Work out the finished part from the listing and answer in its coordinate system (mm). Round coordinates to 2 decimals unless told otherwise and drop trailing zeros. Write each loop counter-clockwise with the first axis right and the second up, starting at its lowest first coordinate (ties: lowest second). Pieces come first, ordered by that corner, then holes.
1. Find section B-B (y = 8.89). Write down the section's boundary in (x, z), and give its area (3 significant figures).
2. Find section A-A (y = -8.89). Write down the section's boundary in (x, z), and give its area (3 significant figures).
3. Determine the mould class of faces 1 (the face through (39.2, -15.4, 0.8)), 2 (the face through (-20.56, -7.94, 4.37)), 3 (the face through (-22, -10, 4.5)) for opening direction X: pulls with the +X half, pulls with the -X half, needs draft (parallel to the pull), parting line crosses it, or undercut.
4. Find section D-D (x = -16). Write down the section's boundary in (y, z), and give its area (3 significant figures).
5. Find section C-C (z = 3.6). Write down the section's boundary in (x, y), and give its area (3 significant figures).
6. A flat-ended cylindrical pin translates along its axis: pin 1 Ø4 at (x, y) = (36.51, -12.7) entering from +Z. Find the tip coordinate at first contact, or state that the pin passes through.
7. Straight lines are drawn through the part: probe 1 along X at (y, z) = (-8.5, 0.4); probe 2 along X at (y, z) = (-9.5, 4.2); probe 3 along Z at (x, y) = (30, -11). For each, find the intervals that lie inside material, in ascending order.
Autodesk Fusion 360 part; units mm, degrees
sketch "Sketch1" plane through (0, 0, 0) normal (0, 0, 1) x (1, 0, 0)
  line L0 (36.5125, -12.7) -> (-36.5125, -12.7) construction
  line L1 (-36.5125, -12.7) -> (-36.5125, 12.7) construction
  line L2 (-36.5125, 12.7) -> (36.5125, 12.7) construction
  line L3 (36.5125, 12.7) -> (36.5125, -12.7) construction
  line L4 (36.5125, -12.7) -> (-36.5125, 12.7) construction
  line L5 (-36.5125, -12.7) -> (36.5125, 12.7) construction
  line L6 (40.3225, -16.51) -> (-40.3225, -16.51)
  line L7 (-40.3225, -16.51) -> (-40.3225, 16.51)
  line L8 (-40.3225, 16.51) -> (40.3225, 16.51)
  line L9 (40.3225, 16.51) -> (40.3225, -16.51)
  circle A0 centre (-36.5125, 12.7) radius 1.524
  circle A1 centre (36.5125, 12.7) radius 1.524
  circle A2 centre (-36.5125, -12.7) radius 1.524
  circle A3 centre (36.5125, -12.7) radius 1.524
  line L10 (22.86, -8.89) -> (-22.86, -8.89) construction
  line L11 (-22.86, -8.89) -> (-22.86, 8.89) construction
  line L12 (-22.86, 8.89) -> (22.86, 8.89) construction
  line L13 (22.86, 8.89) -> (22.86, -8.89) construction
  line L14 (22.86, -8.89) -> (-22.86, 8.89) construction
  line L15 (-22.86, -8.89) -> (22.86, 8.89) construction
  circle A4 centre (-22.86, 8.89) radius 1.143
  circle A5 centre (22.86, 8.89) radius 1.143
  circle A6 centre (-22.86, -8.89) radius 1.143
  circle A7 centre (22.86, -8.89) radius 1.143
  circle A8 centre (-22.86, 8.89) radius 2.413
  circle A9 centre (22.86, 8.89) radius 2.413
  circle A10 centre (-22.86, -8.89) radius 2.413
  circle A11 centre (22.86, -8.89) radius 2.413
  dimension "d1" = 73.025
  dimension "d2" = 25.4
  dimension "d3" = -3.81
  dimension "d4" = 3.048
  dimension "d7" = 73.025
  dimension "d8" = -25.4
  dimension "d9" = 45.72
  dimension "d10" = 17.78
  dimension "d11" = 2.286
  dimension "d14" = 45.72
  dimension "d15" = -17.78
  dimension "d16" = 1.27
  dimension "d17" = 1.27
  dimension "d18" = 1.27
  dimension "d19" = 1.27
extrude "Extrude1" add sketch "Sketch1" along normal blind 1.5 contours L6 L7 L8 L9 | A4 | A8 | A9 | A10 | A11
extrude "Extrude2" add sketch "Sketch1" along normal blind 4.5 contours A9 | A10 | A11
draft "Draft1" angle 30 neutral plane through (0, 0, 4.5) pull (0, 0, 1) 3 faces at (-20.459, -8.6497, 2.5) (25.261, 9.1303, 2.5) (25.261, -8.6497, 2.5)
fillet "Fillet1" radius 3.81 4 edges at (-40.3225, -16.51, 0.75) (-40.3225, 16.51, 0.75) (40.3225, 16.51, 0.75) (40.3225, -16.51, 0.75)
fillet "Fillet2" radius 2 3 edges at (-26.7245, -7.3911, 1.5) (18.9955, -7.3911, 1.5) (18.9955, 10.3889, 1.5)
Worked answers:
1. outline: (-40.32, 0) - (21.72, 0) - (21.72, 4.5) - (20.45, 4.5) - (19.29, 2.5) arc R2 cw to (17.56, 1.5) - (-40.32, 1.5) - close; (24, 0) - (40.32, 0) - (40.32, 1.5) - (28.16, 1.5) arc R2 cw to (26.43, 2.5) - (25.27, 4.5) - (24, 4.5) - close
1. area: 131 mm2
2. outline: (-40.32, 0) - (-24, 0) - (-24, 4.5) - (-25.27, 4.5) - (-26.43, 2.5) arc R2 cw to (-28.16, 1.5) - (-40.32, 1.5) - close; (-21.72, 0) - (21.72, 0) - (21.72, 4.5) - (20.45, 4.5) - (19.29, 2.5) arc R2 cw to (17.56, 1.5) - (-17.56, 1.5) arc R2 cw to (-19.29, 2.5) - (-20.45, 4.5) - (-21.72, 4.5) - close; (24, 0) - (40.32, 0) - (40.32, 1.5) - (28.16, 1.5) arc R2 cw to (26.43, 2.5) - (25.27, 4.5) - (24, 4.5) - close
2. area: 141 mm2
3. face 1: pulls with the +X half
3. face 2: undercut
3. face 3: needs draft
4. outline: (-16.51, 0) - (16.51, 0) - (16.51, 1.5) - (-16.51, 1.5) - close
4. area: 49.5 mm2
5. outline: circle Ø5.87 at (-22.86, -8.89); circle Ø5.87 at (22.86, -8.89); circle Ø5.87 at (22.86, 8.89); hole circle Ø2.29 at (-22.86, -8.89); hole circle Ø2.29 at (22.86, -8.89); hole circle Ø2.29 at (22.86, 8.89)
5. area: 68.7 mm2
6. pin 1: stops at z = 1.5
7. probe 1: x = -40.32 to -23.93, -21.79 to 21.79, 23.93 to 40.32
7. probe 2: x = -25.37 to -23.83, -21.89 to -20.35, 20.35 to 21.89, 23.83 to 25.37
7. probe 3: z = 0 to 1.5
